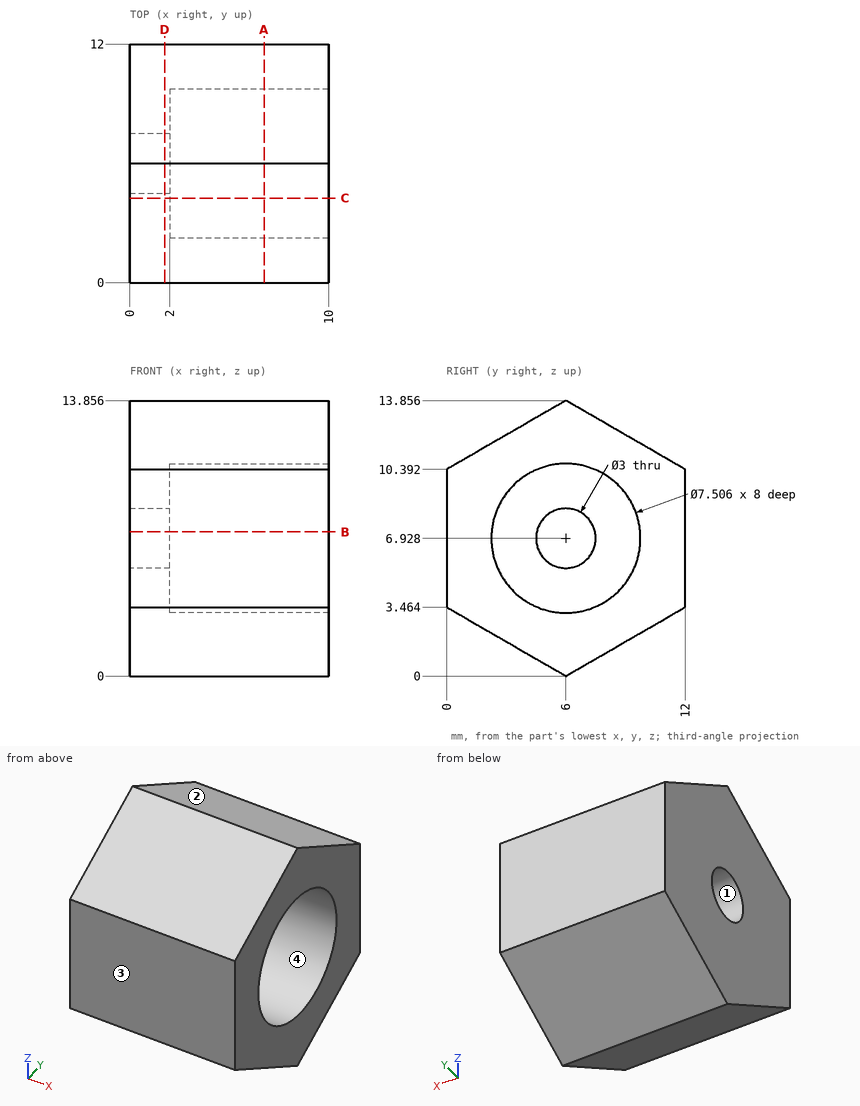
Verification items for this drawing (mm, ordinates from the low corner). Coordinates: 2 decimals unless noted, no trailing zeros. Write each loop counter-clockwise with the first axis right and the second up, starting at its lowest first coordinate (ties: lowest second). Pieces come first, ordered by that corner, then holes. Notation, with made-up numbers: (55.5, 28) -> (59.5, 28) arc R18 cw to (59.5, 41) -> close; hole circle Ø1 at (-28, 75). An arc over 180 degrees is marked (long way). One line per item, written item: value. Start each with the question number.
Q1. Mould release check, pull along Z, two halves, no side actions. Record for the marked faces 1, 2, 3 and 4: pulls with the +Z half, pulls with the -Z half, needs draft (parallel to the pull), parting line crosses it, or undercut.
Q2. Cross-section at A-A on x = 6.75. Enter the section's corners in (y, z) (1 decimal).
Q3. Cross-section at B-B on z = 7.25. Enter the section's corners in (x, y) (1 decimal).
Q4. Go/stop test with flat-tipped pins: P1, Ø6, axis at x = 7.5, y = 9.5, coming from the +Z side; P2, Ø2, axis at y = 1.5, z = 2, coming from the -X side; P3, Ø4.5, axis at y = 6, z = 6.93, coming from the +X side; P4, Ø2, axis at x = 6.5, y = 7.5, coming from the -Z side. Record where each tip stops, or that it passes through.
Q5. Cross-section at C-C on y = 4.25. Enter the section's corners in (x, z).
Q6. Cross-section at D-D on x = 1.75. Enter the section's corners in (y, z) (1 decimal).
Q7. Thickness scan on L1, parallel to X at y = 7, z = 10.5; L2, parallel to Z at x = 5.5, y = 5 (1 decimal); L3, parallel to Z at x = 6.5, y = 3.75 (1 decimal). Record the ranges inside material, lowest first. Write a range as from..to.
Checked values:
1. face 1: undercut
1. face 2: pulls with the +Z half
1. face 3: needs draft
1. face 4: undercut
2. outline: (0, 3.5) -> (6, 0) -> (12, 3.5) -> (12, 10.4) -> (6, 13.9) -> (0, 10.4) -> close; hole circle Ø7.5 at (6, 6.9)
3. outline: (0, 0) -> (10, 0) -> (10, 2.3) -> (2, 2.3) -> (2, 4.5) -> (0, 4.5) -> close; (0, 7.5) -> (2, 7.5) -> (2, 9.7) -> (10, 9.7) -> (10, 12) -> (0, 12) -> close
4. P1: stops at z = 13.57
4. P2: stops at x = 0
4. P3: stops at x = 2
4. P4: stops at z = 0.29
5. outline: (0, 1.01) -> (10, 1.01) -> (10, 3.61) -> (2, 3.61) -> (2, 10.25) -> (10, 10.25) -> (10, 12.85) -> (0, 12.85) -> close
6. outline: (0, 3.5) -> (6, 0) -> (12, 3.5) -> (12, 10.4) -> (6, 13.9) -> (0, 10.4) -> close; hole circle Ø3 at (6, 6.9)
7. L1: x = 0..2
7. L2: z = 0.6..3.3, 10.5..13.3
7. L3: z = 1.3..3.9, 9.9..12.6
